Could you check a few things on this model? Use its own coordinates, in mm. Face numbers are marked on the shaded views. A direction names the side the tool comes from. Coordinates: 2 decimals unless noted, no trailing zeros. Write each loop counter-clockwise with the first axis right and the second up, starting at its lowest first coordinate (ties: lowest second). Pieces come first, ordered by that corner, then holes. Notation, with made-up numbers: M 27.5,61 L 45.5,61 A32 ccw 45.5,99 Z; hole C 3,5 d7. An arc over 180 degrees is marked long. Answer as CSV lines item,"result". Start each with the question number.
Item 1: Suppose I cut it at D-D, the plane y = -13.5. Write out the boundary of the cut face in (x, z) (3 decimals).
Item 2: Suppose I cut it at B-B, the plane y = -6.75. Write out the boundary of the cut face in (x, z) (3 decimals), and give its area (3 significant figures).
Item 3: Suppose I cut it at A-A, the plane x = 0. Write out the boundary of the cut face in (y, z) (3 decimals).
Item 4: If I drill on line 1 along X through (y, z) = (6.75, 3.75); line 2 along Y through (x, z) = (10, 4); line 3 along Y through (x, z) = (12, 3.5), over which ranges is the centre line in solid material (lowest first)? Write a range as [from, to].
Item 5: I'm going to push flat-ended pins straight in: P1, Ø4, axis at x = -12.5, y = -8.5, coming from the -Z side; P2, Ø2, axis at y = -1, z = 1, coming from the -X side; P3, Ø1, axis at y = -12, z = 3, coming from the +X side; P4, Ø1.5, axis at y = 5.5, z = 2.5, coming from the +X side. Where does each tip first touch, or does it pass through?
Item 6: Suppose I cut it at C-C, the plane x = 7. Write out the boundary of the cut face in (y, z) (3 decimals).
Item 7: On a 3-axis mill with a long thin cutter (end or side, diameter ignored), from which of +Z, -Z, +X, -X, +Y, -Y can I reach the whole of each face in a straight line? I mean the marked faces 1 and 2. Say none if no direction works.
Item 8: We'd pull the mould along X, two halves only. Please class the marked faces 3, 4 and 5: +X half, -X half, draft (parallel to the pull), parting line (faces both ways), or undercut.
```python
from build123d import *

# Parameters (mm, degrees)
SKETCH1_R           = 17.5
BOSS_EXTRUDE1_DEPTH = 9.525
SKETCH2_R           = 2.75
M5_THROUGH_DEPTH    = 9.525
SKETCH3_R           = 1.7
M4_DRILL_DEPTH      = 9.525
SKETCH4_R           = 4.25
CUT_EXTRUDE2_DEPTH  = 5


with BuildPart() as part:
    # Sketch1 → Boss-Extrude1 (new body)
    with BuildSketch(Plane.XY):
        with Locations(Location((0, 0, 0), (0, 0, 180))):
            Circle(SKETCH1_R)
    extrude(amount=BOSS_EXTRUDE1_DEPTH)

    # Sketch2 → M5_through (cut)
    with BuildSketch(Plane.XY.offset(9.525)):
        with Locations((0, 13.5)):
            Circle(SKETCH2_R)
        with Locations((11.691342951, 6.75)):
            Circle(SKETCH2_R)
        with Locations((11.691342951, -6.75)):
            Circle(SKETCH2_R)
        with Locations((0, -13.5)):
            Circle(SKETCH2_R)
        with Locations((-11.691342951, -6.75)):
            Circle(SKETCH2_R)
        with Locations((-11.691342951, 6.75)):
            Circle(SKETCH2_R)
    extrude(amount=-M5_THROUGH_DEPTH, mode=Mode.SUBTRACT)

    # Sketch3 → M4_DRILL (cut)
    with BuildSketch(Plane.XY.offset(9.525)):
        with Locations((-3.5, 6.062177826)):
            Circle(SKETCH3_R)
        with Locations((7, 0)):
            Circle(SKETCH3_R)
        with Locations((-3.5, -6.062177826)):
            Circle(SKETCH3_R)
    extrude(amount=-M4_DRILL_DEPTH, mode=Mode.SUBTRACT)

    # Sketch4 → Cut-Extrude2 (cut)
    with BuildSketch(Plane(origin=(0, 0, 0), x_dir=(-1, 0, 0), z_dir=(0, 0, -1))):
        with Locations((0, 13.5)):
            Circle(SKETCH4_R)
        with Locations((11.691342951, 6.75)):
            Circle(SKETCH4_R)
        with Locations((11.691342951, -6.75)):
            Circle(SKETCH4_R)
        with Locations((0, -13.5)):
            Circle(SKETCH4_R)
        with Locations((-11.691342951, -6.75)):
            Circle(SKETCH4_R)
        with Locations((-11.691342951, 6.75)):
            Circle(SKETCH4_R)
    extrude(amount=-CUT_EXTRUDE2_DEPTH, mode=Mode.SUBTRACT)


solid = part.part
```
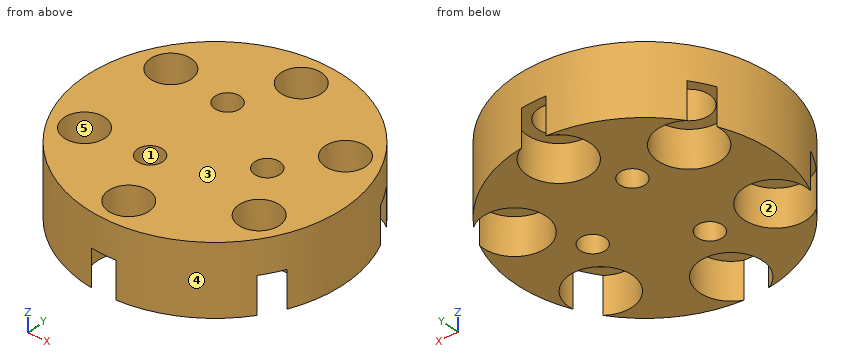
Ans:
1,outline,"M -11.136,0 L -4.25,0 L -4.25,5 L -2.75,5 L -2.75,9.525 L -11.136,9.525 Z; M 2.75,5 L 4.25,5 L 4.25,0 L 11.136,0 L 11.136,9.525 L 2.75,9.525 Z"
2,outline,"M -16.146,0 L -15.941,0 L -15.941,5 L -14.441,5 L -14.441,9.525 L -16.146,9.525 Z; M -8.941,5 L -7.441,5 L -7.441,0 L -5.055,0 L -5.055,9.525 L -8.941,9.525 Z; M -1.945,0 L 7.441,0 L 7.441,5 L 8.941,5 L 8.941,9.525 L -1.945,9.525 Z; M 14.441,5 L 15.941,5 L 15.941,0 L 16.146,0 L 16.146,9.525 L 14.441,9.525 Z"
2,area,"143 mm^2"
3,outline,"M -17.5,5 L -16.25,5 L -16.25,9.525 L -17.5,9.525 Z; M -10.75,5 L -9.25,5 L -9.25,0 L 9.25,0 L 9.25,5 L 10.75,5 L 10.75,9.525 L -10.75,9.525 Z; M 16.25,5 L 17.5,5 L 17.5,9.525 L 16.25,9.525 Z"
4,line 1,"x = [-16.15, -15.94], [-7.44, -5.05], [-1.95, 7.44], [15.94, 16.15]"
4,line 2,"y = [-14.36, -10.65], [-2.85, 2.85], [10.65, 14.36]"
4,line 3,"y = [-12.74, -10.99], [-2.51, 2.51], [10.99, 12.74]"
5,P1,"stops at z = 5"
5,P2,"stops at x = -17.5"
5,P3,"stops at x = 13.19"
5,P4,"stops at x = 16.84"
6,outline,"M -16.039,0 L -1.7,0 L -1.7,9.525 L -16.039,9.525 Z; M 1.7,0 L 16.039,0 L 16.039,9.525 L 1.7,9.525 Z"
7,face 1,"+Z, -Z"
7,face 2,"-Z"
8,face 3,"draft"
8,face 4,"parting line"
8,face 5,"undercut"
